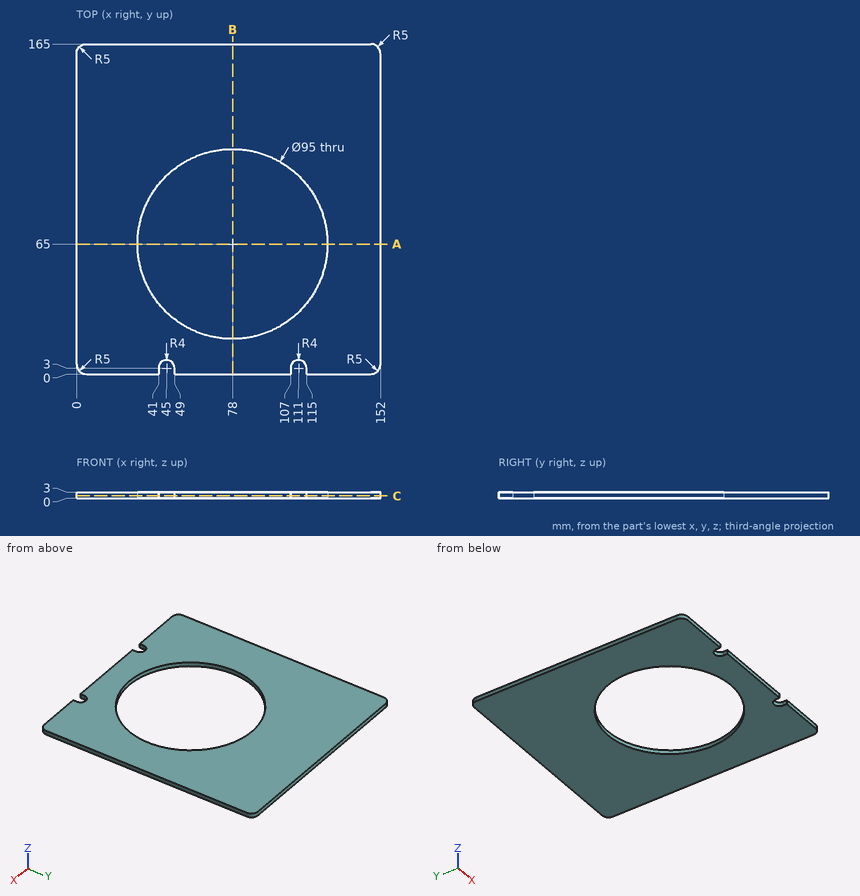
Verification items for this drawing (mm, ordinates from the low corner). Round coordinates to 2 decimals unless told otherwise and drop trailing zeros. Write each loop counter-clockwise with the first axis right and the second up, starting at its lowest first coordinate (ties: lowest second). Pieces come first, ordered by that corner, then holes. Notation, with made-up numbers: (49.25, 0.25) - (80.25, 0.25) arc R18 cw to (80.25, 13.25) - close; hole circle Ø8 at (19, -20). An arc over 180 degrees is marked (long way). Answer as a JSON object with one key per item and string values. Group by question number.
Q1. Section check C-C, the plane z = 1.05. Enter the section's corners in (x, y).
Q2. Section check A-A, the plane y = 65. Enter the section's corners in (x, z).
Q3. Go/stop test with flat-tipped pins: pin 1 Ø1 at (y, z) = (98, 0.5) entering from -X; pin 2 Ø1.5 at (y, z) = (2, 2) entering from +X. Record where each tip stops, or that it passes through.
Q4. Section check B-B, the plane x = 78. Enter the section's corners in (y, z).
Q5. Thickness scan on line 1 (Y direction, x = 78, z = 1.35); line 2 (Y direction, x = 113, z = 0.7); line 3 (X direction, y = 60, z = 1.25). Record the ranges inside material, lowest first.
Found:
{
 "1": {"outline": "(0, 5) arc R5 ccw to (5, 0) - (41, 0) - (41, 3) arc R4 cw to (49, 3) - (49, 0) - (107, 0) - (107, 3) arc R4 cw to (115, 3) - (115, 0) - (147, 0) arc R5 ccw to (152, 5) - (152, 160) arc R5 ccw to (147, 165) - (5, 165) arc R5 ccw to (0, 160) - close; hole circle Ø95 at (78, 65)"},
 "2": {"outline": "(0, 0) - (30.5, 0) - (30.5, 3) - (0, 3) - close; (125.5, 0) - (152, 0) - (152, 3) - (125.5, 3) - close"},
 "3": {"pin 1": "stops at x = 0", "pin 2": "stops at x = 151.47"},
 "4": {"outline": "(0, 0) - (17.5, 0) - (17.5, 3) - (0, 3) - close; (112.5, 0) - (165, 0) - (165, 3) - (112.5, 3) - close"},
 "5": {"line 1": "y = 0 to 17.5, 112.5 to 165", "line 2": "y = 6.46 to 32.89, 97.11 to 165", "line 3": "x = 0 to 30.76, 125.24 to 152"}
}
